Geometry: final body of the model. Coordinates: model frame, mm. A direction names the side the tool comes from. Give positions to 0.01 mm unless a question says otherwise; leave off trailing zeros. Order: outer loops, then holes, each group sorted by start corner. A loop starts at its lowest first (then second) coordinate and runs counter-clockwise, first axis right, second up. Notation, with made-up numbers: (-15.5, 42) - (28.5, 42) arc R27 cw to (28.5, 69) - close; hole circle Ø4 at (45, 58.25). An arc over 180 degrees is marked (long way). Use one line per item in the form item = value.
from build123d import *

# Parameters (mm, degrees)
PAD004_DEPTH    = 30
THICKNESS_T     = 1.3
SKETCH008_R     = 15
POCKET002_DEPTH = 5
SKETCH010_W     = 4
SKETCH010_H     = 4
SKETCH010_R     = 1.4
PAD006_DEPTH    = 10
POCKET003_DEPTH = 5
SKETCH013_R     = 6
POCKET004_DEPTH = 5


with BuildPart() as part:
    # CopySketch007 → Pad004 (new body, symmetric)
    with BuildSketch(Plane.XY):
        Polygon((5, 0), (5, 16.3299316186), (-48.4572350855, 27.2418440368), (-78.9897948557, 27.2418440368), (-78.9897948557, 0), align=None)
    extrude(amount=PAD004_DEPTH, both=True)

    # Thickness
    thickness_openings = [part.faces().sort_by_distance(p)[0] for p in [
        (-36.994897, 0, 0),
    ]]
    offset(amount=THICKNESS_T, openings=thickness_openings)

    # Sketch008 (on Face24 of Thickness) → Pocket002 (cut)
    with BuildSketch(Plane(origin=(3.66, 17.9302649172, 0), x_dir=(-0.9797958971, 0.2, 0), z_dir=(0.2, 0.9797958971, 0))):
        with Locations((23.2739585094, 7.9084926401)):
            Circle(SKETCH008_R)
    extrude(amount=-POCKET002_DEPTH, mode=Mode.SUBTRACT)

    # Sketch010 (on Face17 of Pocket002) → Pad006 (join)
    with BuildSketch(Plane.XZ):
        with Locations((-76.9897948557, 28)):
            Rectangle(SKETCH010_W, SKETCH010_H)
        with Locations((-76.9897948557, 28)):
            Circle(SKETCH010_R, mode=Mode.SUBTRACT)
        with Locations((-76.9897948557, -28)):
            Rectangle(SKETCH010_W, SKETCH010_H)
        with Locations((-76.9897948557, -28)):
            Circle(SKETCH010_R, mode=Mode.SUBTRACT)
        with Locations((3, -28)):
            Rectangle(SKETCH010_W, SKETCH010_H)
        with Locations((3, -28)):
            Circle(SKETCH010_R, mode=Mode.SUBTRACT)
        with Locations((3, 28)):
            Rectangle(SKETCH010_W, SKETCH010_H)
        with Locations((3, 28)):
            Circle(SKETCH010_R, mode=Mode.SUBTRACT)
    extrude(amount=-PAD006_DEPTH)

    # Sketch012 (on Face8 of Pad006) → Pocket003 (cut)
    with BuildSketch(Plane.XY.offset(31.3)):
        with BuildLine():
            ThreePointArc((-67.0672858986, 15.4269435951), (-70.0672858986, 12.4269435951), (-67.0672858986, 9.4269435951))
            Line((-67.0672858986, 9.4269435951), (-52.0672858986, 9.4269435951))
            ThreePointArc((-52.0672858986, 9.4269435951), (-49.0672858986, 12.4269435951), (-52.0672858986, 15.4269435951))
            Line((-67.0672858986, 15.4269435951), (-52.0672858986, 15.4269435951))
        make_face()
    extrude(amount=-POCKET003_DEPTH, mode=Mode.SUBTRACT)

    # Sketch013 (on Face25 of Pocket003) → Pocket004 (cut)
    with BuildSketch(Plane(origin=(0, 0, -31.3), x_dir=(1, 0, 0), z_dir=(0, 0, -1))):
        with Locations((-31.571347, -11.873986)):
            Circle(SKETCH013_R)
    extrude(amount=-POCKET004_DEPTH, mode=Mode.SUBTRACT)


solid = part.part
(1) Ray query, line 1 along Z through (x, y) = (3, 5.5); line 2 along Z through (x, y) = (-29, 20.5); line 3 along Z through (x, y) = (1.5, 7). Return the intervals inside material, ascending.
Computed values:
line_1 = -31.3 to -29.4, -26.6 to -26, 26 to 26.6, 29.4 to 31.3
line_2 = -31.3 to -30, 30 to 31.3
line_3 = -31.3 to -26, 26 to 31.3
(2) Contact query for flat-ended pins moving along their axis: pin 1 Ø3 at (x, z) = (3, 28.5) entering from +Y; pin 2 Ø2 at (x, y) = (-32, 9) entering from -Z; pin 3 Ø1 at (x, z) = (-37.5, 13) entering from -Y. Output: stop coordinate, or through.
Computed values:
pin_1 = 18.37
pin_2 = 30
pin_3 = 24.9
(3) Cut plane B-B on x = -62. Output: boundary loops of the cut face in (y, z), plus the area to 3 significant figures.
Computed values:
outline = (0, -31.3) - (27.24, -31.3) arc R1.3 ccw to (28.54, -30) - (28.54, 30) arc R1.3 ccw to (27.24, 31.3) - (15.43, 31.3) - (15.43, 30) - (27.24, 30) - (27.24, -30) - (0, -30) - close; (0, 30) - (9.43, 30) - (9.43, 31.3) - (0, 31.3) - close
area = 144 mm²
(4) Cut plane C-C on y = 2.5. Output: boundary loops of the cut face in (x, z).
Computed values:
outline = (-80.29, -30) arc R1.3 ccw to (-78.99, -31.3) - (5, -31.3) arc R1.3 ccw to (6.3, -30) - (6.3, 30) arc R1.3 ccw to (5, 31.3) - (-78.99, 31.3) arc R1.3 ccw to (-80.29, 30) - close; hole (-78.99, -26) - (-74.99, -26) - (-74.99, -30) - (1, -30) - (1, -26) - (5, -26) - (5, 26) - (1, 26) - (1, 30) - (-74.99, 30) - (-74.99, 26) - (-78.99, 26) - close; hole circle Ø2.8 at (-76.99, -28); hole circle Ø2.8 at (-76.99, 28); hole circle Ø2.8 at (3, -28); hole circle Ø2.8 at (3, 28)
(5) Pull-direction query (Z, two-part tool) for faces 6 (the face through (-25.85, 10.07, -30.66)), 7 (the face through (-38, 14, 30)), 8 (the face through (-21.92, 22.75, 30.93)), 9 (the face through (-78.4, 10, 28.9)); classes: released by +Z, released by -Z, zero draft, split by the parting line, or undercut.
Computed values:
face_6 = zero draft
face_7 = undercut
face_8 = released by +Z
face_9 = undercut
(6) Cut plane D-D on y = 14.25. Output: boundary loops of the cut face in (x, z).
Computed values:
outline = (-80.29, -30) arc R1.3 ccw to (-78.99, -31.3) - (-37.08, -31.3) - (-37.08, -30) - (-78.99, -30) - (-78.99, 30) - (-69.45, 30) - (-69.45, 31.3) - (-78.99, 31.3) arc R1.3 ccw to (-80.29, 30) - close; (-49.68, 30) - (5, 30) - (5, -30) - (-26.06, -30) - (-26.06, -31.3) - (5, -31.3) arc R1.3 ccw to (6.3, -30) - (6.3, 30) arc R1.3 ccw to (5, 31.3) - (-49.68, 31.3) - close
(7) Cut plane A-A on z = 28. Output: boundary loops of the cut face in (x, y).
Computed values:
outline = (-80.29, 0) - (-78.39, 0) - (-78.39, 10) - (-78.99, 10) - (-78.99, 27.24) - (-48.46, 27.24) - (5, 16.33) - (5, 10) - (4.4, 10) - (4.4, 0) - (6.3, 0) - (6.3, 16.33) arc R1.3 ccw to (5.26, 17.6) - (-48.2, 28.52) arc R1.3 ccw to (-48.46, 28.54) - (-78.99, 28.54) arc R1.3 ccw to (-80.29, 27.24) - close; (-75.59, 0) - (-74.99, 0) - (-74.99, 10) - (-75.59, 10) - close; (1, 0) - (1.6, 0) - (1.6, 10) - (1, 10) - close
(8) Reachability of faces 1 (the face through (1, 5, -28)), 2 (the face through (1.6, 10, -27.1)), 3 (the face through (-34, 0, 30.3)), 4 (the face through (-70.067, 12.493, 30.659)), 5 (the face through (-38, 14, 31.3)) from +Z, -Z, +X, -X, +Y, -Y: full face, straight path, thin tool, end or side. Return the list, or none.
Computed values:
face_1 = -Y
face_2 = none
face_3 = +Z, -Z, +X, -X, -Y
face_4 = +Z
face_5 = +Z, +X, -X, +Y, -Y
